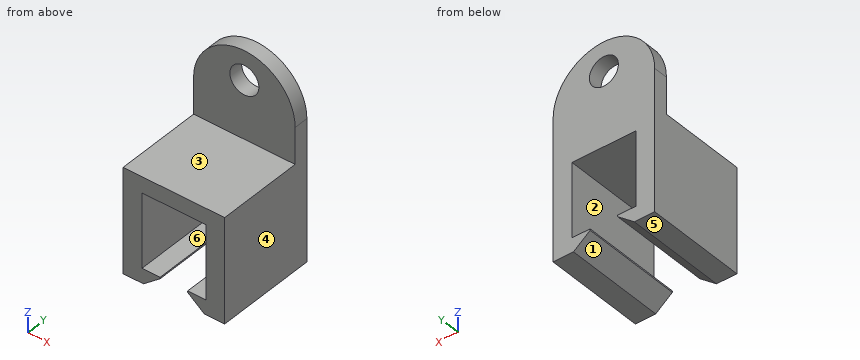
```python
from build123d import *

# Parameters (mm, degrees)
F1_DEPTH = 7
F0_R     = 1
F2_DEPTH = 1


with BuildPart() as f1:
    # F0 (on Front) → F1 (new body)
    with BuildSketch(Plane.XZ):
        Polygon((-0.95, -6.2), (-2.2, -6.2), (-2.2, -1.1), (2.2, -1.1), (2.2, -6.2), (0.95, -6.2), (0.95, -6.3), (2.094895, -7.2), (3.5, -7.2), (3.5, 0), (-3.5, 0), (-3.5, -7.2), (-2.094895, -7.2), (-0.95, -6.3), align=None)
    extrude(amount=F1_DEPTH)

    # F0 (on Front) → F2 (join)
    with BuildSketch(Plane.XZ):
        with BuildLine():
            Line((-3.5, 2.5), (-3.5, 0))
            Line((-3.5, 0), (3.5, 0))
            Line((3.5, 0), (3.5, 2.5))
            ThreePointArc((3.5, 2.5), (0, 6), (-3.5, 2.5))
        make_face()
        with Locations((0, 4)):
            Circle(F0_R, mode=Mode.SUBTRACT)
    extrude(amount=F2_DEPTH)


solid = f1.part
```
Here's how the part is built. I have some questions about the finished solid (model axes, mm). Face numbers are marked on the shaded views. A direction names the side the tool comes from. Coordinates: 2 decimals unless noted, no trailing zeros. Loops run counter-clockwise (first coordinate to the right, second up) from the corner with the lowest first, then second, coordinate; pieces in that order, holes last. Notation, with made-up numbers: M 76,23 L 116,23 A31 cw 116,57 Z; hole C -20.75,35.25 d7. An arc over 180 degrees is marked long. One line per item, written item: value.
1. Imagine slicing it at D-D (y = -1.75). List the corners of the cut face in (x, z) for me.
Geometry says:
outline: M -3.5,-7.2 L -2.09,-7.2 L -0.95,-6.3 L -0.95,-6.2 L -2.2,-6.2 L -2.2,-1.1 L 2.2,-1.1 L 2.2,-6.2 L 0.95,-6.2 L 0.95,-6.3 L 2.09,-7.2 L 3.5,-7.2 L 3.5,0 L -3.5,0 Z
2. Will these pins go through, and if not, where does the flat tip stop? pin 1 Ø0.6 at (x, y) = (-1.5, -2.5) entering from +Z; pin 2 Ø1.3 at (x, y) = (0.5, -2.5) entering from -Z; pin 3 Ø1.5 at (x, z) = (-1, 2.5) entering from -Y.
Geometry says:
pin 1: stops at z = 0
pin 2: stops at z = -6.46
pin 3: stops at y = -1
3. Please list where these lines run through material, in increasing order: probe 1 along X at (y, z) = (-1.5, -3); probe 2 along Z at (x, y) = (0, -0.2); probe 3 along X at (y, z) = (-2.75, -6.25).
Geometry says:
probe 1: x = -3.5 to -2.2, 2.2 to 3.5
probe 2: z = -1.1 to 3, 5 to 6
probe 3: x = -3.5 to -0.95, 0.95 to 3.5
4. On a 3-axis mill with a long thin cutter (end or side, diameter ignored), from which of +Z, -Z, +X, -X, +Y, -Y can I reach the whole of each face in a straight line? I mean the marked faces 1, 2 and 3. Say none if no direction works.
Geometry says:
face 1: -Z, +Y, -Y
face 2: +Y, -Y
face 3: +Z, +X, -X, -Y
5. Imagine slicing it at A-A (x = 0). List the corners of the cut face in (y, z) for me.
Geometry says:
outline: M -7,-1.1 L 0,-1.1 L 0,3 L -1,3 L -1,0 L -7,0 Z; M -1,5 L 0,5 L 0,6 L -1,6 Z
6. Imagine slicing it at C-C (y = -0.25). List the corners of the cut face in (x, z) for me.
Geometry says:
outline: M -3.5,-7.2 L -2.09,-7.2 L -0.95,-6.3 L -0.95,-6.2 L -2.2,-6.2 L -2.2,-1.1 L 2.2,-1.1 L 2.2,-6.2 L 0.95,-6.2 L 0.95,-6.3 L 2.09,-7.2 L 3.5,-7.2 L 3.5,2.5 A3.5 ccw -3.5,2.5 Z; hole C 0,4 d2
7. Imagine slicing it at B-B (z = -1.5). List the corners of the cut face in (x, y) for me.
Geometry says:
outline: M -3.5,-7 L -2.2,-7 L -2.2,0 L -3.5,0 Z; M 2.2,-7 L 3.5,-7 L 3.5,0 L 2.2,0 Z
8. Thinking about a two-plate mould opening in X: for the marked faces 4, 5 and 6, which applies, +X half, -X half, draft (parallel to the pull), parting line (faces both ways), or undercut?
Geometry says:
face 4: +X half
face 5: draft
face 6: undercut
